Could you check a few things on this model? Use its own coordinates, in mm. Face numbers are marked on the shaded views. Round coordinates to 2 decimals unless told otherwise and drop trailing zeros. Write each loop counter-clockwise with the first axis right and the second up, starting at its lowest first coordinate (ties: lowest second). Pieces come first, ordered by that corner, then holes. Notation, with made-up numbers: (46, 68.25) - (92, 68.25) arc R20 cw to (92, 100.25) - close; hole circle Ø3 at (62.5, 35.5). An arc over 180 degrees is marked (long way). Write each question's results on one line, items separated by ' | '. Start each with the question number.
(1) Imagine slicing it at A-A on x = 0. Write out the boundary of the cut face in (y, z) (1 decimal).
(2) Thinking about a two-plate mould opening in Y: for the marked faces 1, 2, 3 and 4, which applies, +Y half, -Y half, draft (parallel to the pull), parting line (faces both ways), or undercut?
(3) Imagine slicing it at B-B on y = 0. Write out the boundary of the cut face in (x, z) (3 decimals), then the cut area to 3 significant figures.
(4) Imagine slicing it at C-C on z = 6.25. Write out the boundary of the cut face in (x, y).
(5) Please list where these lines run through material, in increasing order: line 1 (Y direction, x = 0, z = 4); line 2 (Y direction, x = 39.5, z = 1.75); line 3 (X direction, y = -22.5, z = 14.75). Write a range as [from, to].
(6) Imagine slicing it at D-D on y = -43.5. Write out the boundary of the cut face in (x, z) (3 decimals).
(7) For P1, Ø7, axis at x = 37.17, y = 21.46, coming from the -Z side, with a flat end and sliding along its axis, tell me the tip position at first contact or that it passes through.
Autodesk Inventor part; units mm, degrees
ref_plane "YZ Plane" through (0, 0, 0) normal (1, 0, 0) x (0, 1, 0)
ref_plane "XZ Plane" through (0, 0, 0) normal (0, 1, 0) x (-1, 0, 0)
ref_plane "XY Plane" through (0, 0, 0) normal (0, 0, 1) x (1, 0, 0)
sketch "Sketch1" plane through (0, 0, 0) normal (0, 0, 1) x (1, 0, 0)
  line L0 (88.9, -88.9) -> (-88.9, -88.9)
  line L1 (-88.9, -88.9) -> (-88.9, 88.9)
  line L2 (-88.9, 88.9) -> (88.9, 88.9)
  line L3 (88.9, 88.9) -> (88.9, -88.9)
  line L4 (88.9, -88.9) -> (-88.9, 88.9) construction
  line L5 (-88.9, -88.9) -> (88.9, 88.9) construction
  point P0 (0, 0)
  dimension "d2" = 177.8
extrude "Extrusion1" add sketch "Sketch1" along normal blind 15.875
sketch "Sketch2" plane through (0, 0, 0) normal (0, 0, -1) x (-1, 0, 0)
  circle A0 centre (0, 0) radius 60.325
  circle A1 centre (0, 42.9196) radius 9.6774
  circle A2 centre (-37.1695, 21.4598) radius 9.6774
  circle A3 centre (-37.1695, -21.4598) radius 9.6774
  circle A4 centre (0, -42.9196) radius 9.6774
  circle A5 centre (37.1695, -21.4598) radius 9.6774
  circle A6 centre (37.1695, 21.4598) radius 9.6774
  line L0 (18.829, -36.4227) -> (14.1966, -28.3993)
  arc A7 (-14.1966, -28.3993) -> (14.1966, -28.3993) centre (0, 0) ccw
  line L1 (-14.1966, -28.3993) -> (-18.829, -36.4227)
  line L2 (-18.829, -36.4227) -> (-22.1285, -34.5177)
  line L3 (-22.1285, -34.5177) -> (-17.4962, -26.4943)
  arc A8 (-31.6928, -1.905) -> (-17.4962, -26.4943) centre (0, 0) ccw
  line L4 (-31.6928, -1.905) -> (-40.9575, -1.905)
  line L5 (-40.9575, -1.905) -> (-40.9575, 1.905)
  line L6 (-40.9575, 1.905) -> (-31.6928, 1.905)
  arc A9 (-17.4962, 26.4943) -> (-31.6928, 1.905) centre (0, 0) ccw
  line L7 (-17.4962, 26.4943) -> (-22.1285, 34.5177)
  line L8 (-22.1285, 34.5177) -> (-18.829, 36.4227)
  line L9 (-18.829, 36.4227) -> (-14.1966, 28.3993)
  arc A10 (14.1966, 28.3993) -> (-14.1966, 28.3993) centre (0, 0) ccw
  line L10 (14.1966, 28.3993) -> (18.829, 36.4227)
  line L11 (18.829, 36.4227) -> (22.1285, 34.5177)
  line L12 (22.1285, 34.5177) -> (17.4962, 26.4943)
  arc A11 (31.6928, 1.905) -> (17.4962, 26.4943) centre (0, 0) ccw
  line L13 (31.6928, 1.905) -> (40.9575, 1.905)
  line L14 (40.9575, 1.905) -> (40.9575, -1.905)
  line L15 (40.9575, -1.905) -> (31.6928, -1.905)
  arc A12 (17.4962, -26.4943) -> (31.6928, -1.905) centre (0, 0) ccw
  line L16 (17.4962, -26.4943) -> (22.1285, -34.5177)
  line L17 (22.1285, -34.5177) -> (18.829, -36.4227)
  point P0 (0, 0)
hole "Hole1" at (0, 42.9196, 0) at (37.1695, 21.4598, 0) at (37.1695, -21.4598, 0) at (0, -42.9196, 0) at (-37.1695, -21.4598, 0) at (-37.1695, 21.4598, 0) direction (0, 0, 1) diameter 7.7978 end through all
sketch "Sketch3" plane through (0, 0, 15.875) normal (0, 0, 1) x (1, 0, 0)
  circle A0 centre (0, 0) radius 20.6375
  point P0 (0, 0)
hole "Hole2" at (0, 0, 15.875) direction (0, 0, -1) diameter 50.8 end through all
properties part number "Mounting Plate" material "Aluminum 6061"
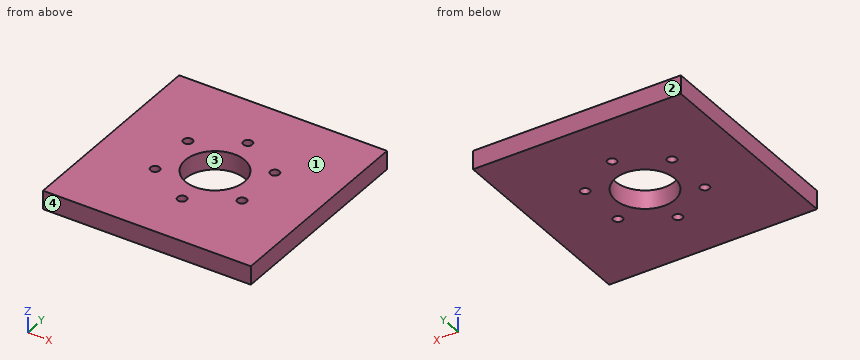
Response:
1) outline: (-88.9, 0) - (-46.8, 0) - (-46.8, 15.9) - (-88.9, 15.9) - close; (-39, 0) - (-25.4, 0) - (-25.4, 15.9) - (-39, 15.9) - close; (25.4, 0) - (39, 0) - (39, 15.9) - (25.4, 15.9) - close; (46.8, 0) - (88.9, 0) - (88.9, 15.9) - (46.8, 15.9) - close
2) face 1: draft | face 2: +Y half | face 3: undercut | face 4: -Y half
3) outline: (-88.9, 0) - (-25.4, 0) - (-25.4, 15.875) - (-88.9, 15.875) - close; (25.4, 0) - (88.9, 0) - (88.9, 15.875) - (25.4, 15.875) - close | area: 2,020 mm²
4) outline: (-88.9, -88.9) - (88.9, -88.9) - (88.9, 88.9) - (-88.9, 88.9) - close; hole circle Ø7.8 at (-37.17, -21.46); hole circle Ø7.8 at (-37.17, 21.46); hole circle Ø50.8 at (0, 0); hole circle Ø7.8 at (0, -42.92); hole circle Ø7.8 at (0, 42.92); hole circle Ø7.8 at (37.17, -21.46); hole circle Ø7.8 at (37.17, 21.46)
5) line 1: [-88.9, -46.82], [-39.02, -25.4], [25.4, 39.02], [46.82, 88.9] | line 2: [-88.9, -24.59], [-18.33, 18.33], [24.59, 88.9] | line 3: [-88.9, -40.93], [-33.41, -11.79], [11.79, 33.41], [40.93, 88.9]
6) outline: (-88.9, 0) - (-3.855, 0) - (-3.855, 15.875) - (-88.9, 15.875) - close; (3.855, 0) - (88.9, 0) - (88.9, 15.875) - (3.855, 15.875) - close
7) P1: through
